from build123d import *

# Parameters (mm, degrees)
SKETCH1_R           = 93.6625
BOSS_EXTRUDE1_DEPTH = 12.7
SKETCH2_R           = 54.102
CUT_EXTRUDE1_DEPTH  = 13.7
SKETCH3_R           = 63.5
CUT_EXTRUDE2_DEPTH  = 2.54
SKETCH4_R           = 2.54
CUT_EXTRUDE3_DEPTH  = 13.7
CIRPATTERN1_COUNT   = 12
SKETCH5_R           = 88.9
SKETCH5_R_2         = 85.725
CUT_EXTRUDE4_DEPTH  = 3.175


with BuildPart() as part:
    # Sketch1 → Boss-Extrude1 (new body)
    with BuildSketch(Plane(origin=(0, 0, 0), x_dir=(1, 0, 0), z_dir=(0, 1, 0))):
        Circle(SKETCH1_R)
    extrude(amount=BOSS_EXTRUDE1_DEPTH)

    # Sketch2 → Cut-Extrude1 (cut, through all)
    with BuildSketch(Plane(origin=(0, 12.7, 0), x_dir=(1, 0, 0), z_dir=(0, 1, 0))):
        Circle(SKETCH2_R)
    extrude(amount=-CUT_EXTRUDE1_DEPTH, mode=Mode.SUBTRACT)

    # Sketch3 → Cut-Extrude2 (cut)
    with BuildSketch(Plane(origin=(0, 12.7, 0), x_dir=(1, 0, 0), z_dir=(0, 1, 0))):
        Circle(SKETCH3_R)
    extrude(amount=-CUT_EXTRUDE2_DEPTH, mode=Mode.SUBTRACT)

    # Sketch4 → Cut-Extrude3 (cut, through all)
    with BuildSketch(Plane(origin=(0, 12.7, 0), x_dir=(1, 0, 0), z_dir=(0, 1, 0))):
        with Locations((0, 58.42)):
            Circle(SKETCH4_R)
    cut_extrude3 = extrude(amount=-CUT_EXTRUDE3_DEPTH, mode=Mode.SUBTRACT)

    # CirPattern1: Cut-Extrude3 ×12 about axis
    cirpattern1_axis = Axis((0, 0, 0), (0, 1, 0))
    for i in range(1, CIRPATTERN1_COUNT):
        add(cut_extrude3.rotate(cirpattern1_axis, i * 360 / CIRPATTERN1_COUNT), mode=Mode.SUBTRACT)

    # Sketch5 → Cut-Extrude4 (cut)
    with BuildSketch(Plane(origin=(0, 12.7, 0), x_dir=(1, 0, 0), z_dir=(0, 1, 0))):
        Circle(SKETCH5_R)
        Circle(SKETCH5_R_2, mode=Mode.SUBTRACT)
    extrude(amount=-CUT_EXTRUDE4_DEPTH, mode=Mode.SUBTRACT)


solid = part.part
Could you check a few things on this model? Use its own coordinates, in mm. A direction names the side the tool comes from. Round coordinates to 2 decimals unless told otherwise and drop trailing zeros. Loops run counter-clockwise (first coordinate to the right, second up) from the corner with the lowest first, then second, coordinate; pieces in that order, holes last. Notation, with made-up numbers: (-18, 42) - (10, 42) arc R17 cw to (10, 61) - close; hole circle Ø7 at (-1, 39.5). An arc over 180 degrees is marked (long way). Write item = value, one per line.
1) Imagine slicing it at B-B (z = 0). Please give me the cut outline in (x, y) (1 decimal).
Computed:
outline = (-93.7, 0) - (-61, 0) - (-61, 10.2) - (-63.5, 10.2) - (-63.5, 12.7) - (-85.7, 12.7) - (-85.7, 9.5) - (-88.9, 9.5) - (-88.9, 12.7) - (-93.7, 12.7) - close; (-55.9, 0) - (-54.1, 0) - (-54.1, 10.2) - (-55.9, 10.2) - close; (54.1, 0) - (55.9, 0) - (55.9, 10.2) - (54.1, 10.2) - close; (61, 0) - (93.7, 0) - (93.7, 12.7) - (88.9, 12.7) - (88.9, 9.5) - (85.7, 9.5) - (85.7, 12.7) - (63.5, 12.7) - (63.5, 10.2) - (61, 10.2) - close
2) If we mould it in two halves opening along X, with no side actions, what happens to faces 3 (the cylindrical face through (-0.55, 5.15, -55.94)), 4 (the flat face through (-64, 12.7, 0)), 5 (the cylindrical face through (89.34, 6.26, -28.13))? For each: pulls with the +X half, pulls with the -X half, needs draft (parallel to the pull), parting line crosses it, or undercut.
Computed:
face_3 = undercut
face_4 = needs draft
face_5 = parting line crosses it
3) Imagine slicing it at A-A (x = 0). Please give me the cut outline in (y, z) (1 decimal), and give its area (3 significant figures).
Computed:
outline = (0, -93.7) - (12.7, -93.7) - (12.7, -88.9) - (9.5, -88.9) - (9.5, -85.7) - (12.7, -85.7) - (12.7, -63.5) - (10.2, -63.5) - (10.2, -61) - (0, -61) - close; (0, -55.9) - (10.2, -55.9) - (10.2, -54.1) - (0, -54.1) - close; (0, 54.1) - (10.2, 54.1) - (10.2, 55.9) - (0, 55.9) - close; (0, 61) - (10.2, 61) - (10.2, 63.5) - (12.7, 63.5) - (12.7, 85.7) - (9.5, 85.7) - (9.5, 88.9) - (12.7, 88.9) - (12.7, 93.7) - (0, 93.7) - close
area = 834 mm2
4) On a 3-axis mill with a long thin cutter (end or side, diameter ignored), from which of +Z, -Z, +X, -X, +Y, -Y can I reach the whole of each face in a straight line? I mean faces 1 (the cylindrical face through (30.76, 5.15, -48.58)), 2 (the cylindrical face through (46.09, 11.13, -72.28)). Say none if no direction works.
Computed:
face_1 = +Y, -Y
face_2 = +Y
5) Imagine slicing it at D-D (z = 58.42). Please give me the cut outline in (x, y) (3 decimals), and give its area (3 significant figures).
Computed:
outline = (-73.21, 0) - (-2.54, 0) - (-2.54, 10.16) - (-24.887, 10.16) - (-24.887, 12.7) - (-62.737, 12.7) - (-62.737, 9.525) - (-67.01, 9.525) - (-67.01, 12.7) - (-73.21, 12.7) - close; (2.54, 0) - (73.21, 0) - (73.21, 12.7) - (67.01, 12.7) - (67.01, 9.525) - (62.737, 9.525) - (62.737, 12.7) - (24.887, 12.7) - (24.887, 10.16) - (2.54, 10.16) - close
area = 1,650 mm2
6) I need wall thicknesses on line 1 along Z through (x, y) = (0, 11) (1 decimal); line 2 along X through (y, z) = (11.25, 65.5); line 3 along X through (y, z) = (5.25, -29.21). Which ranges of each line are inside material? Lowest first, please. Write a range as from..to.
Computed:
line_1 = -93.7..-88.9, -85.7..-63.5, 63.5..85.7, 88.9..93.7
line_2 = -66.95..-60.11, -55.3..55.3, 60.11..66.95
line_3 = -88.99..-53.13, -48.05..-45.54, 45.54..48.05, 53.13..88.99
7) I'm going to push flat-ended pins straight in: P1, Ø8, axis at x = 30, z = 48.5, coming from the +Y side; P2, Ø4.5, axis at x = -29.21, z = 50.59, coming from the +Y side; P3, Ø2, axis at x = -40.5, y = 9.5, coming from the +Z side; P4, Ø4, axis at y = 8.5, z = -19, coming from the +X side. Where does each tip first touch, or does it pass through?
Computed:
P1 = 10.16
P2 = through
P3 = 84.93
P4 = 92.11
8) Imagine slicing it at C-C (y = 3.75). Give the number of separate pieces and of enclosed holes in the cut face, and give its area (3 significant figures).
Computed:
separate_pieces = 1
enclosed_holes = 13
area = 18,100 mm2
